Could you check a few things on this drawing? It's one solid part, dimensions in mm from its lowest x, y, z. A direction names the side the tool comes from. Give positions to 0.01 mm unless a question says otherwise; leave off trailing zeros. Order: outer loops, then holes, each group sorted by start corner. A loop starts at its lowest first (then second) coordinate and runs counter-clockwise, first axis right, second up. Notation, with made-up numbers: (-3, 42) -> (55, 42) arc R14 cw to (55, 56) -> close; hole circle Ø8 at (-20.75, 42). An arc over 180 degrees is marked (long way). Answer as CSV lines item,"result".
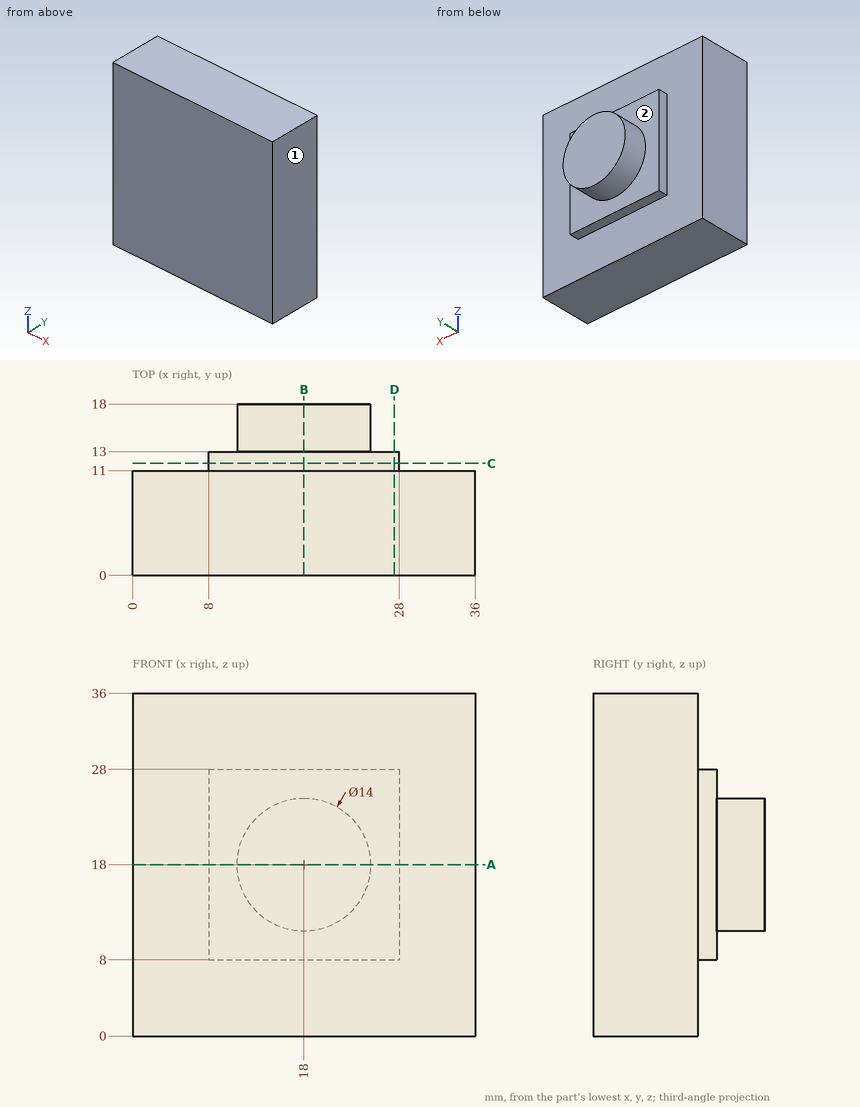
Item 1: Please list where these lines run through material, in increasing order: line 1 along Y through (x, z) = (20, 7); line 2 along Y through (x, z) = (8.5, 27.5); line 3 along Z through (x, y) = (8.5, 11.5).
Numbers:
line 1,"y = 0 to 11"
line 2,"y = 0 to 13"
line 3,"z = 8 to 28"
Item 2: Imagine slicing it at D-D, the plane x = 27.5. Please give me the cut outline in (y, z), then the cut area to 3 significant figures.
Numbers:
outline,"(0, 0) -> (11, 0) -> (11, 8) -> (13, 8) -> (13, 28) -> (11, 28) -> (11, 36) -> (0, 36) -> close"
area,"436 mm²"
Item 3: Imagine slicing it at C-C, the plane y = 11.75. Please give me the cut outline in (x, z), then the cut area to 3 significant figures.
Numbers:
outline,"(8, 8) -> (28, 8) -> (28, 28) -> (8, 28) -> close"
area,"400 mm²"
Item 4: For the marked faces 1 and 2, which set-ups out of +Z, -Z, +X, -X, +Y, -Y let a thin tool reach every point of the face, with its end or its side?
Numbers:
face 1,"+Z, -Z, +X, +Y, -Y"
face 2,"+Y"
Item 5: Imagine slicing it at A-A, the plane z = 18. Please give me the cut outline in (x, y), then the cut area to 3 significant figures.
Numbers:
outline,"(0, 0) -> (36, 0) -> (36, 11) -> (28, 11) -> (28, 13) -> (25, 13) -> (25, 18) -> (11, 18) -> (11, 13) -> (8, 13) -> (8, 11) -> (0, 11) -> close"
area,"506 mm²"
Item 6: Imagine slicing it at B-B, the plane x = 18. Please give me the cut outline in (y, z), then the cut area to 3 significant figures.
Numbers:
outline,"(0, 0) -> (11, 0) -> (11, 8) -> (13, 8) -> (13, 11) -> (18, 11) -> (18, 25) -> (13, 25) -> (13, 28) -> (11, 28) -> (11, 36) -> (0, 36) -> close"
area,"506 mm²"
Item 7: For pin 1 (12 mm diameter, centred on x = 28.5, z = 13, fed in from -Y); pin 2 (1.6 mm diameter, centred on y = 12, z = 16, fed in from +X); pin 3 (1 mm diameter, centred on x = 17.5, y = 12, fed in from -Z); pin 4 (6 mm diameter, centred on x = 23.5, z = 6.5, fed in from +Y), each with a flat end and sliding along its axis, tell me the tip position at first contact or that it passes through.
Numbers:
pin 1,"stops at y = 0"
pin 2,"stops at x = 28"
pin 3,"stops at z = 8"
pin 4,"stops at y = 13"
